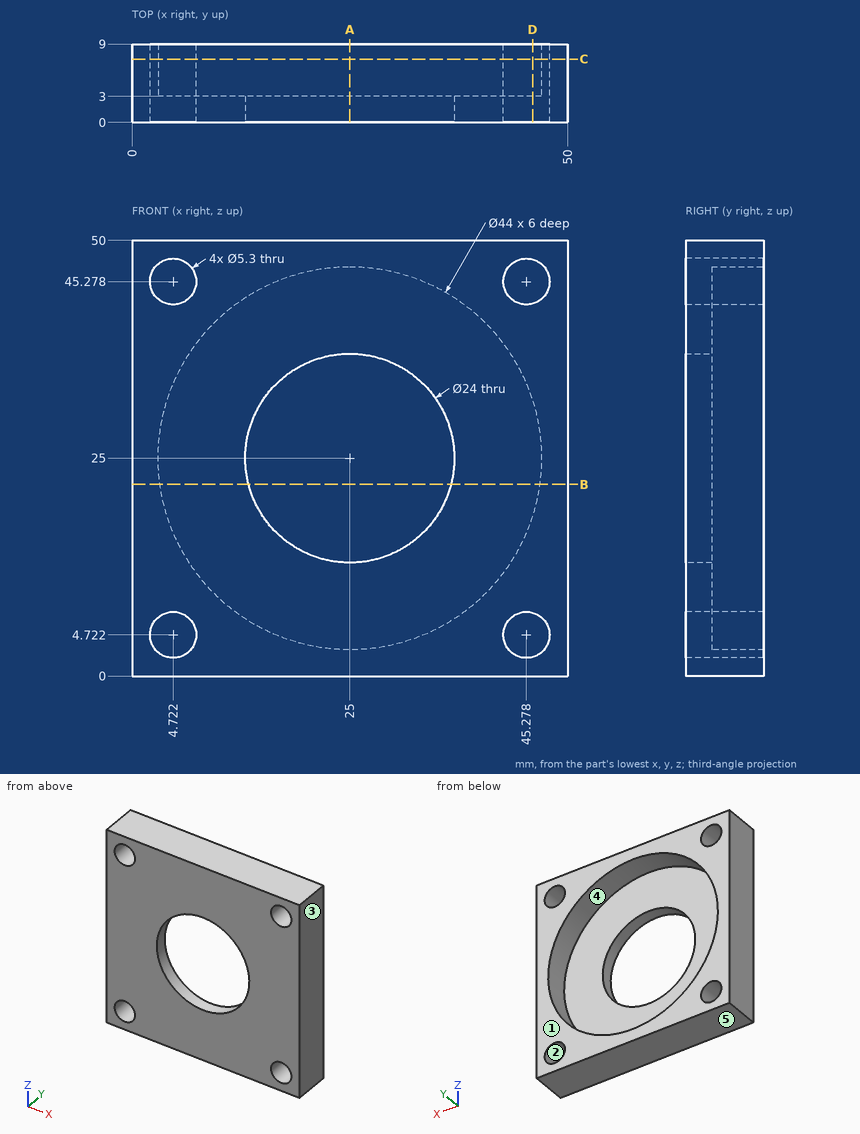
The drawing under review shows one solid part. Ordinate dimensions are in mm from its lowest x, y, z. A direction names the side the tool comes from. Coordinates: 2 decimals unless noted, no trailing zeros. Order: outer loops, then holes, each group sorted by start corner. A loop starts at its lowest first (then second) coordinate and runs counter-clockwise, first axis right, second up. Notation, with made-up numbers: (78.5, 5.25) -> (105.5, 5.25) arc R36 ccw to (105.5, 43.25) -> close; hole circle Ø7 at (24, 32). An arc over 180 degrees is marked (long way). One line per item, written item: value.
1) We need section B-B, the plane z = 22. Give the boundary of the cut face in (x, y), then the cut area to 3 significant figures.
Output values:
outline: (0, 0) -> (13.38, 0) -> (13.38, 3) -> (3.21, 3) -> (3.21, 9) -> (0, 9) -> close; (36.62, 0) -> (50, 0) -> (50, 9) -> (46.79, 9) -> (46.79, 3) -> (36.62, 3) -> close
area: 119 mm2
2) We need section D-D, the plane x = 46. Give the boundary of the cut face in (y, z).
Output values:
outline: (0, 0) -> (9, 0) -> (9, 2.17) -> (0, 2.17) -> close; (0, 7.27) -> (9, 7.27) -> (9, 18.44) -> (3, 18.44) -> (3, 31.56) -> (9, 31.56) -> (9, 42.73) -> (0, 42.73) -> close; (0, 47.83) -> (9, 47.83) -> (9, 50) -> (0, 50) -> close
3) To check wall thickness, follow probe 1 along Z at (x, y) = (25.5, 4); probe 2 along X at (y, z) = (0.5, 30); probe 3 along X at (y, z) = (4, 9). State the ranges of each line that lie inside material, in increasing order. Write a range as [from, to].
Output values:
probe 1: z = [0, 3.01], [46.99, 50]
probe 2: x = [0, 14.09], [35.91, 50]
probe 3: x = [0, 9.9], [40.1, 50]
4) Clearance check with a flat-ended pin moving along its axis: P1, Ø4, axis at x = 9, z = 21, coming from the +Y side. State where the tip first meets the part, or that it passes through.
Output values:
P1: stops at y = 3
5) We need section C-C, the plane y = 7.25. Give the boundary of the cut face in (x, z).
Output values:
outline: (0, 0) -> (50, 0) -> (50, 50) -> (0, 50) -> close; hole circle Ø5.3 at (4.72, 4.72); hole circle Ø5.3 at (4.72, 45.28); hole circle Ø44 at (25, 25); hole circle Ø5.3 at (45.28, 4.72); hole circle Ø5.3 at (45.28, 45.28)
6) Machinability: for the marked faces 4 and 5, which of the approach directions +Z, -Z, +X, -X, +Y, -Y give a long, thin tool a straight path to every point of the face, cutting with its end or side? Answer none if there is none.
Output values:
face 4: +Y
face 5: -Z, +X, -X, +Y, -Y
7) We need section A-A, the plane x = 25. Give the boundary of the cut face in (y, z), then the cut area to 3 significant figures.
Output values:
outline: (0, 0) -> (9, 0) -> (9, 3) -> (3, 3) -> (3, 13) -> (0, 13) -> close; (0, 37) -> (3, 37) -> (3, 47) -> (9, 47) -> (9, 50) -> (0, 50) -> close
area: 114 mm2
8) Draft analysis for pull direction X (two halves, no side actions). For the marked faces 1, 2 and 3, state which applies: +X half, -X half, draft (parallel to the pull), parting line (faces both ways), or undercut.
Output values:
face 1: draft
face 2: undercut
face 3: +X half
